```python
from build123d import *

# Parameters (mm, degrees)
SKETCH_1_R      = 1.6
EXTRUDE_1_DEPTH = 3


with BuildPart() as part:
    # 草图1 → 凸台-拉伸1 (new body)
    # profile 1 of 2: a face of its own
    with BuildSketch(Plane.XY):
        with BuildLine():
            Line((0, 27.154799922), (0, 35.904799922))
            Line((0, 35.904799922), (-18, 35.904799922))
            ThreePointArc((-18, 35.904799922), (-20.121320344, 35.026120265), (-21, 32.904799922))
            Line((-21, 32.904799922), (-21, -23.095200078))
            ThreePointArc((-21, -23.095200078), (-20.121320344, -25.216520422), (-18, -26.095200078))
            Line((-18, -26.095200078), (0, -26.095200078))
            Line((0, -26.095200078), (0, 2.654799922))
            ThreePointArc((0, 2.654799922), (-12.25, 14.904799922), (0, 27.154799922))
        make_face()
        with BuildLine():
            ThreePointArc((-10, -16.495200078), (-12.5, -18.995200078), (-15, -16.495200078))
            Line((-15, -16.495200078), (-15, -15.695200078))
            ThreePointArc((-15, -15.695200078), (-12.5, -13.195200078), (-10, -15.695200078))
            Line((-10, -15.695200078), (-10, -16.495200078))
        make_face(mode=Mode.SUBTRACT)
        with Locations((-15.5, -0.595200078)):
            Circle(SKETCH_1_R, mode=Mode.SUBTRACT)
        with Locations((-15.5, 30.404799922)):
            Circle(SKETCH_1_R, mode=Mode.SUBTRACT)
    # profile 2 of 2: a face of its own
    with BuildSketch(Plane.XY):
        with BuildLine():
            Line((18, 35.904799922), (0, 35.904799922))
            Line((0, 35.904799922), (0, 27.154799922))
            ThreePointArc((0, 27.154799922), (8.66205807, 23.566857991), (12.25, 14.904799922))
            ThreePointArc((12.25, 14.904799922), (8.66205807, 6.242741852), (0, 2.654799922))
            Line((0, 2.654799922), (0, -26.095200078))
            Line((0, -26.095200078), (18, -26.095200078))
            ThreePointArc((18, -26.095200078), (20.121320344, -25.216520422), (21, -23.095200078))
            Line((21, -23.095200078), (21, 32.904799922))
            ThreePointArc((21, 32.904799922), (20.121320344, 35.026120265), (18, 35.904799922))
        make_face()
        with BuildLine():
            Line((15, -15.695200078), (15, -16.495200078))
            ThreePointArc((15, -16.495200078), (12.5, -18.995200078), (10, -16.495200078))
            Line((10, -16.495200078), (10, -15.695200078))
            ThreePointArc((10, -15.695200078), (12.5, -13.195200078), (15, -15.695200078))
        make_face(mode=Mode.SUBTRACT)
        with Locations((15.5, -0.595200078)):
            Circle(SKETCH_1_R, mode=Mode.SUBTRACT)
        with Locations((15.5, 30.404799922)):
            Circle(SKETCH_1_R, mode=Mode.SUBTRACT)
    extrude(amount=EXTRUDE_1_DEPTH)


solid = part.part
```
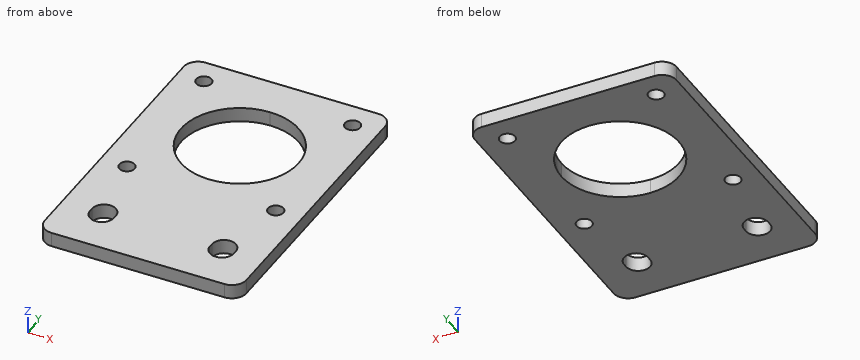
The listing builds one solid part. Answer for the finished solid, in the listing's coordinates (mm). Coordinates: 2 decimals unless noted, no trailing zeros. Write each loop counter-clockwise with the first axis right and the second up, starting at its lowest first coordinate (ties: lowest second). Pieces come first, ordered by that corner, then holes.
Q1. Section C-C, the plane z = 0.7 is taken. Write down the section's boundary in (x, y), then the cut area to 3 significant figures.
Returned:
outline: (-21, -23.1) arc R3 ccw to (-18, -26.1) - (18, -26.1) arc R3 ccw to (21, -23.1) - (21, 32.9) arc R3 ccw to (18, 35.9) - (-18, 35.9) arc R3 ccw to (-21, 32.9) - close; hole circle Ø3.2 at (-15.5, -0.6); hole circle Ø3.2 at (-15.5, 30.4); hole (-15, -16.5) arc R2.5 ccw to (-10, -16.5) - (-10, -15.7) arc R2.5 ccw to (-15, -15.7) - close; hole circle Ø24.5 at (0, 14.9); hole (10, -16.5) arc R2.5 ccw to (15, -16.5) - (15, -15.7) arc R2.5 ccw to (10, -15.7) - close; hole circle Ø3.2 at (15.5, -0.6); hole circle Ø3.2 at (15.5, 30.4)
area: 2,050 mm2
Q2. Section A-A, the plane x = 8.5 is taken. Write down the section's boundary in (y, z), then the cut area to 3 significant figures.
Returned:
outline: (-26.1, 0) - (6.08, 0) - (6.08, 3) - (-26.1, 3) - close; (23.73, 0) - (35.9, 0) - (35.9, 3) - (23.73, 3) - close
area: 133 mm2
Q3. Find the intervals of material crossed by line 1 along Y through (x, z) = (-15.5, 2.1); line 2 along X through (y, z) = (22, 1.05); line 3 along X through (y, z) = (10, 2.8), in increasing order.
Returned:
line 1: y = -26.1 to -2.2, 1 to 28.8, 32 to 35.9
line 2: x = -21 to -9.99, 9.99 to 21
line 3: x = -21 to -11.23, 11.23 to 21
Q4. Section B-B, the plane y = 22 is taken. Write down the section's boundary in (x, z), then the cut area to 3 significant figures.
Returned:
outline: (-21, 0) - (-9.99, 0) - (-9.99, 3) - (-21, 3) - close; (9.99, 0) - (21, 0) - (21, 3) - (9.99, 3) - close
area: 66.1 mm2
Q5. Given P1, Ø5, axis at x = 15.5, y = -0.6, coming from the +Z side, flat-ended and moving along its own axis, determine where the tip first touches the part or whether it passes through.
Returned:
P1: stops at z = 3
